Build history of the part. All positions in model axes, mm. Give positions to 0.01 mm unless a question says otherwise; leave off trailing zeros. Loops run counter-clockwise (first coordinate to the right, second up) from the corner with the lowest first, then second, coordinate; pieces in that order, holes last. Notation, with made-up numbers: (52, -25) -> (98, -25) arc R10 ccw to (98, -8) -> close; hole circle Ø10 at (22, -34). An arc over 180 degrees is marked (long way). One line per question, with ' | ' between items. Start each with the question number.
(1) Slice it at C-C, the plane z = 0.5. Give the number of separate pieces and of enclosed holes in the cut face, then the cut area to 3 significant figures.
(2) Slice it at B-B, the plane x = -31.5. Write the cut outline in (y, z), then the cut area to 3 significant figures.
(3) Slice it at A-A, the plane y = -20. Write the cut outline in (x, z).
(4) Drill centre lines: L1, parallel to X at y = -24, z = 0.45; L2, parallel to Y at x = 21.5, z = 1.1; L3, parallel to X at y = -38.5, z = 2.05. Where is each one in solid material? Low to high. Write a range as from..to.
(5) Flat gauge pins, fed straight in: pin 1 Ø3.5 at (x, y) = (93.66, -38.1) entering from +Z; pin 2 Ø7 at (x, y) = (-93.66, 38.1) entering from +Z. Where does each tip first touch, or does it go through?
(6) Slice it at D-D, the plane y = 24.5. Write the cut outline in (x, z), then the cut area to 3 significant figures.
```python
from build123d import *

# Parameters (mm, degrees)
SKETCH_W   = 203.2
SKETCH_H   = 88.9
SKETCH_R   = 2.775
SKETCH_W_2 = 130.302
SKETCH_H_2 = 43.9
SKETCH_W_3 = 18
SKETCH_H_3 = 25
PAD_DEPTH  = 2.2


with BuildPart() as part:
    # Sketch → Pad (new body)
    with BuildSketch(Plane.XY):
        Rectangle(SKETCH_W, SKETCH_H)
        with Locations((-93.6625, 38.1)):
            Circle(SKETCH_R, mode=Mode.SUBTRACT)
        with Locations((-93.6625, -38.1)):
            Circle(SKETCH_R, mode=Mode.SUBTRACT)
        with Locations((93.6625, 38.1)):
            Circle(SKETCH_R, mode=Mode.SUBTRACT)
        with Locations((93.6625, -38.1)):
            Circle(SKETCH_R, mode=Mode.SUBTRACT)
        with Locations((0, 14.5)):
            Rectangle(SKETCH_W_2, SKETCH_H_2, mode=Mode.SUBTRACT)
        with Locations((48.151, -23.95)):
            Rectangle(SKETCH_W_3, SKETCH_H_3, mode=Mode.SUBTRACT)
        with Locations((22.151, -23.95)):
            Rectangle(SKETCH_W_3, SKETCH_H_3, mode=Mode.SUBTRACT)
    extrude(amount=PAD_DEPTH)


solid = part.part
```
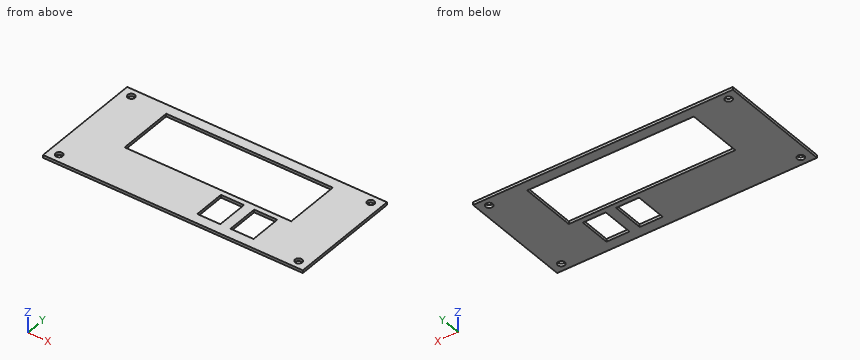
Final values:
1) separate pieces: 1 | enclosed holes: 7 | area: 11,300 mm2
2) outline: (-44.45, 0) -> (-7.45, 0) -> (-7.45, 2.2) -> (-44.45, 2.2) -> close; (36.45, 0) -> (44.45, 0) -> (44.45, 2.2) -> (36.45, 2.2) -> close | area: 99.0 mm2
3) outline: (-101.6, 0) -> (13.15, 0) -> (13.15, 2.2) -> (-101.6, 2.2) -> close; (31.15, 0) -> (39.15, 0) -> (39.15, 2.2) -> (31.15, 2.2) -> close; (57.15, 0) -> (101.6, 0) -> (101.6, 2.2) -> (57.15, 2.2) -> close
4) L1: -101.6..13.15, 31.15..39.15, 57.15..101.6 | L2: -44.45..-36.45, -11.45..-7.45, 36.45..44.45 | L3: -101.6..-96.41, -90.92..90.92, 96.41..101.6
5) pin 1: through | pin 2: z = 2.2
6) outline: (-101.6, 0) -> (-65.15, 0) -> (-65.15, 2.2) -> (-101.6, 2.2) -> close; (65.15, 0) -> (101.6, 0) -> (101.6, 2.2) -> (65.15, 2.2) -> close | area: 160 mm2
